Input: part model. Units: mm. Frame: model coordinates. Round coordinates to 2 decimals unless told otherwise and drop trailing zeros. Loops run counter-clockwise (first coordinate to the right, second up) from the corner with the lowest first, then second, coordinate; pieces in that order, holes last. Notation, with made-up numbers: M -19.75,-10.5 L -8.75,-10.5 A25 ccw -8.75,9.5 Z; hole C 49,17.25 d1. An arc over 180 degrees is marked long. Use one line per item in the form item = value. Start each with the question number.
Q1. Ray query, line 1 along Z through (x, y) = (-41, 0.15); line 2 along Z through (x, y) = (0, -0.15). Return the intervals inside material, ascending.
Q2. Section query A-A, the plane z = -41. Output: boundary loops of the cut face in (x, y), and give its area (3 significant figures).
Q3. Section query C-C, the plane y = -0.25. State how many separate pieces and enclosed holes the cut face has, and give its area (3 significant figures).
Q4. Section query B-B, the plane x = 0. Output: boundary loops of the cut face in (y, z), and give its area (3 significant figures).
Q5. Section query D-D, the plane x = 41. Output: boundary loops of the cut face in (y, z), and give its area (3 significant figures).
```python
from build123d import *

# Parameters (mm, degrees)
SKETCH1_W               = 92
SKETCH1_H               = 92
BOSS_EXTRUDE1_DEPTH     = 0.5
FILLET1_R               = 2
CUT_EXTRUDE1_DEPTH      = 66.061509358
CUT_EXTRUDE1_DEPTH_BACK = 66.061509358
SKETCH2_R               = 3


with BuildPart() as part:
    # Sketch1 → Boss-Extrude1 (new, symmetric)
    with BuildSketch(Plane(origin=(0, 0, 0), x_dir=(1, 0, 0), z_dir=(0, 1, 0))):
        Rectangle(SKETCH1_W, SKETCH1_H)
    extrude(amount=BOSS_EXTRUDE1_DEPTH, both=True)

    # Fillet1
    fillet1_edges = [part.edges().sort_by_distance(p)[0] for p in [
        (46, 0, 46),
        (-46, 0, 46),
        (-46, 0, -46),
        (46, 0, -46),
    ]]
    fillet(fillet1_edges, radius=FILLET1_R)

    # Sketch2 → Cut-Extrude1 (cut, two sides: drawn at the far end of the back side and taken through both)
    with BuildSketch(Plane(origin=(0, 0.5, 0), x_dir=(1, 0, 0), z_dir=(0, 1, 0)).offset(-CUT_EXTRUDE1_DEPTH_BACK)):
        with Locations(Location((-41, 41, 0), (0, 0, 270))):
            Circle(SKETCH2_R)
        with Locations(Location((0, 41, 0), (0, 0, 270))):
            Circle(SKETCH2_R)
        with Locations(Location((41, 41, 0), (0, 0, 270))):
            Circle(SKETCH2_R)
        with Locations(Location((41, 0, 0), (0, 0, 270))):
            Circle(SKETCH2_R)
        with Locations(Location((41, -41, 0), (0, 0, 270))):
            Circle(SKETCH2_R)
        with Locations(Location((0, -41, 0), (0, 0, 270))):
            Circle(SKETCH2_R)
        with Locations(Location((-41, -41, 0), (0, 0, 270))):
            Circle(SKETCH2_R)
        with Locations(Location((-41, 0, 0), (0, 0, 270))):
            Circle(SKETCH2_R)
    extrude(amount=CUT_EXTRUDE1_DEPTH + CUT_EXTRUDE1_DEPTH_BACK, mode=Mode.SUBTRACT)


solid = part.part
```
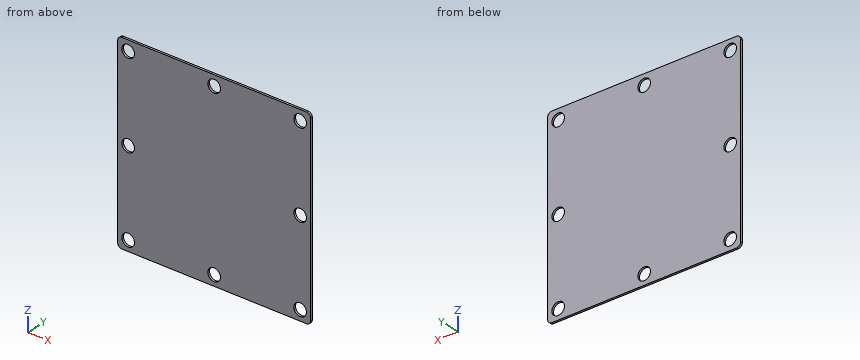
Results found:
q1.line_1 = -46 to -44, -38 to -3, 3 to 38, 44 to 46
q1.line_2 = -46 to -44, -38 to 38, 44 to 46
q2.outline = M -46,-0.5 L -44,-0.5 L -44,0.5 L -46,0.5 Z; M -38,-0.5 L -3,-0.5 L -3,0.5 L -38,0.5 Z; M 3,-0.5 L 38,-0.5 L 38,0.5 L 3,0.5 Z; M 44,-0.5 L 46,-0.5 L 46,0.5 L 44,0.5 Z
q2.area = 74.0 mm²
q3.separate_pieces = 1
q3.enclosed_holes = 8
q3.area = 8,230 mm²
q4.outline = M -0.5,-46 L 0.5,-46 L 0.5,-44 L -0.5,-44 Z; M -0.5,-38 L 0.5,-38 L 0.5,38 L -0.5,38 Z; M -0.5,44 L 0.5,44 L 0.5,46 L -0.5,46 Z
q4.area = 80.0 mm²
q5.outline = M -0.5,-46 L 0.5,-46 L 0.5,-44 L -0.5,-44 Z; M -0.5,-38 L 0.5,-38 L 0.5,-3 L -0.5,-3 Z; M -0.5,3 L 0.5,3 L 0.5,38 L -0.5,38 Z; M -0.5,44 L 0.5,44 L 0.5,46 L -0.5,46 Z
q5.area = 74.0 mm²
